Autodesk Inventor part; units mm, degrees
ref_plane "YZ Plane" through (0, 0, 0) normal (1, 0, 0) x (0, 1, 0)
ref_plane "XZ Plane" through (0, 0, 0) normal (0, 1, 0) x (-1, 0, 0)
ref_plane "XY Plane" through (0, 0, 0) normal (0, 0, 1) x (1, 0, 0)
sketch "Sketch1" plane through (0, 0, 0) normal (0, 1, 0) x (-1, 0, 0)
  line L0 (0, 0) -> (-50.8, 0)
  line L1 (-50.8, 0) -> (-50.8, -25.4)
  line L2 (-50.8, -25.4) -> (0, -25.4)
  line L3 (0, -25.4) -> (0, 0)
  line L4 (-3.175, -22.225) -> (-47.625, -22.225)
  line L5 (-47.625, -22.225) -> (-47.625, -3.175)
  line L6 (-47.625, -3.175) -> (-3.175, -3.175)
  line L7 (-3.175, -3.175) -> (-3.175, -22.225)
  dimension "d0" = 50.8
  dimension "d1" = 25.4
  dimension "d2" = 3.175
  dimension "d3" = 3.175
  dimension "d4" = 3.175
  dimension "d5" = 3.175
extrude "Extrusion1" add sketch "Sketch1" along normal blind 660.4
sketch "Sketch2" plane through (0, 0, 0) normal (0, 0, 1) x (1, 0, 0)
  line L0 (3.175, 660.4) -> (47.625, 660.4)
  line L1 (25.4, 660.4) -> (25.4, 0)
  line L2 (25.4, 0) -> (25.4, 330.2)
  line L3 (25.4, 330.2) -> (22.225, 330.2)
  circle A0 centre (22.225, 330.2) radius 14.2875
  point P0 (0, 0)
  dimension "d11" = 3.175
extrude "Extrusion2" cut sketch "Sketch2" against normal blind 25.4
sketch "Sketch3" plane through (0, 0, 0) normal (0, 0, 1) x (1, 0, 0)
  line L0 (0, 0) -> (50.8, 0)
  line L1 (25.4, 0) -> (25.4, 660.4)
  line L2 (0, 660.4) -> (50.8, 660.4)
  line L3 (25.4, 660.4) -> (25.4, 571.5)
  line L4 (25.4, 0) -> (25.4, 88.9)
  line L5 (25.4, 571.5) -> (25.4, 555.625)
  circle A0 centre (25.4, 555.625) radius 14.2875
  line L6 (25.4, 88.9) -> (25.4, 104.775)
  circle A1 centre (25.4, 104.775) radius 14.2875
  dimension "d12" = 88.9
  dimension "d13" = 88.9
  dimension "d17" = 15.875
  dimension "d18" = 15.875
extrude "Extrusion3" cut sketch "Sketch3" against normal blind 25.4
properties part number "26in 2x1" material "Aluminum 6061"
Could you check a few things on this model? Use its own coordinates, in mm. A direction names the side the tool comes from. Give positions to 0.01 mm unless a question says otherwise; leave off trailing zeros. Order: outer loops, then holes, each group sorted by start corner. A loop starts at its lowest first (then second) coordinate and runs counter-clockwise, first axis right, second up. Notation, with made-up numbers: (-29.5, 13.25) -> (8.5, 13.25) arc R17 cw to (8.5, 32.25) -> close; hole circle Ø2 at (77, 89.5). An arc over 180 degrees is marked (long way). Answer in a Markdown table with one row per item. Add a question column.
Item 1: Imagine slicing it at B-B (y = 330.2). List the corners of the cut face in (x, z) for me (1 decimal), and give its area (3 significant figures).
Item 2: For faces 1 (the flat face through (47.625, 326, -13)), 2 (the flat face through (26, 0, -2)), which set-ups out of +Z, -Z, +X, -X, +Y, -Y let a thin tool reach every point of the face, with its end or its side?
Item 3: Please list where these lines run through material, in increasing order: probe 1 along Z at (x, y) = (17, 162.5) (3 decimals); probe 2 along X at (y, z) = (103, -21.5) (3 decimals); probe 3 along Y at (x, z) = (25.4, -1.65).
Item 4: Imagine slicing it at D-D (x = 21). Count the separate pieces of the cut face and the enclosed holes in it, and give its area (3 significant figures).
Item 5: We'd pull the mould along Z, two halves only. Please class faces 3 (the flat face through (37, 326, -25.4)), 4 (the flat face through (36.3, 325.6, 0)), 5 (the flat face through (40, 326, -22.225)), 6 (the cylindrical face through (22.303, 541.677, -1.565)): pulls with the +Z half, pulls with the -Z half, needs draft (parallel to the pull), parting line crosses it, or undercut.
Item 6: Imagine slicing it at A-A (z = -16.5). List the corners of the cut face in (x, y) for me (3 decimals).
Item 7: Imagine slicing it at C-C (y = 84). List the corners of the cut face in (x, z) for me (3 decimals), and give its area (3 significant figures).
Item 8: I'm going to push flat-ended pins straight in: P1, Ø1.5, axis at x = 7, y = 336.5, coming from the +Z side; P2, Ø23, axis at x = 22.225, y = 330.2, coming from the -Z side. Where does each tip first touch, or does it pass through?
Result:
| question | item | result |
|---|---|---|
| 1 | outline | (0, -25.4) -> (7.9, -25.4) -> (7.9, -22.2) -> (3.2, -22.2) -> (3.2, -3.2) -> (7.9, -3.2) -> (7.9, 0) -> (0, 0) -> close; (36.5, -25.4) -> (50.8, -25.4) -> (50.8, 0) -> (36.5, 0) -> (36.5, -3.2) -> (47.6, -3.2) -> (47.6, -22.2) -> (36.5, -22.2) -> close |
| 1 | area | 262 mm2 |
| 2 | face 1 | +Y, -Y |
| 2 | face 2 | +Z, -Z, +X, -X, -Y |
| 3 | probe 1 | -25.4 to -22.225, -3.175 to 0 |
| 3 | probe 2 | 0 to 3.175, 47.625 to 50.8 |
| 3 | probe 3 | 0 to 90.49, 119.06 to 316.27, 344.13 to 541.34, 569.91 to 660.4 |
| 4 | separate pieces | 8 |
| 4 | enclosed holes | 0 |
| 4 | area | 3,670 mm2 |
| 5 | face 3 | pulls with the -Z half |
| 5 | face 4 | pulls with the +Z half |
| 5 | face 5 | undercut |
| 5 | face 6 | needs draft |
| 6 | outline | (0, 0) -> (3.175, 0) -> (3.175, 660.4) -> (0, 660.4) -> close; (47.625, 0) -> (50.8, 0) -> (50.8, 660.4) -> (47.625, 660.4) -> close |
| 7 | outline | (0, -25.4) -> (50.8, -25.4) -> (50.8, 0) -> (0, 0) -> close; hole (3.175, -22.225) -> (47.625, -22.225) -> (47.625, -3.175) -> (3.175, -3.175) -> close |
| 7 | area | 444 mm2 |
| 8 | P1 | z = 0 |
| 8 | P2 | through |
